Study the drawing (mm; zero at the part's minimum x, y, z) and answer. Coordinates: 2 decimals unless noted, no trailing zeros. Order: outer loops, then holes, each group sorted by start corner. A loop starts at its lowest first (then second) coordinate and runs counter-clockwise, first axis right, second up. Notation, with made-up numbers: (26, -9.75) - (56, -9.75) arc R29 ccw to (56, 26.25) - close; hole circle Ø10 at (51, 51.25). An arc over 180 degrees is marked (long way). Write item = value, one per line.
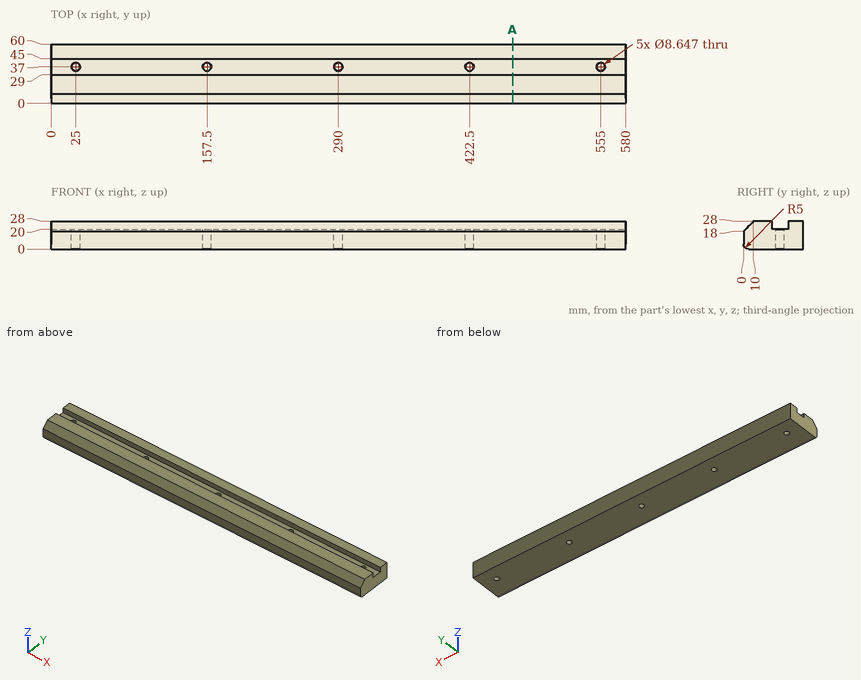
1) Flat-ended cylindrical pins translate along their axes: pin 1 Ø8 at (x, y) = (346.5, 34) entering from +Z; pin 2 Ø6.5 at (x, z) = (432.5, 22.5) entering from -Y; pin 3 Ø5 at (x, y) = (290, 37) entering from -Z. Find the tip coordinate at first contact, or state that the pin passes through.
Returned:
pin_1 = 20
pin_2 = 1.25
pin_3 = through
2) Straight lines are drawn through the part: line 1 along X through (y, z) = (37, 6.75); line 2 along Y through (x, z) = (157.5, 12.25); line 3 along Y through (x, z) = (510.5, 26.75). For each, find the intervals that lie inside material, in ascending order. Write a range as from..to.
Returned:
line_1 = 0..20.68, 29.32..153.18, 161.82..285.68, 294.32..418.18, 426.82..550.68, 559.32..580
line_2 = 0..32.68, 41.32..60
line_3 = 8.75..29, 45..60
3) The part is cut by section A-A (x = 466). Determine the outline of the cut face in (y, z).
Returned:
outline = (0, 5) arc R5 ccw to (5, 0) - (60, 0) - (60, 28) - (45, 28) - (45, 20) - (29, 20) - (29, 28) - (10, 28) - (0, 18) - close
